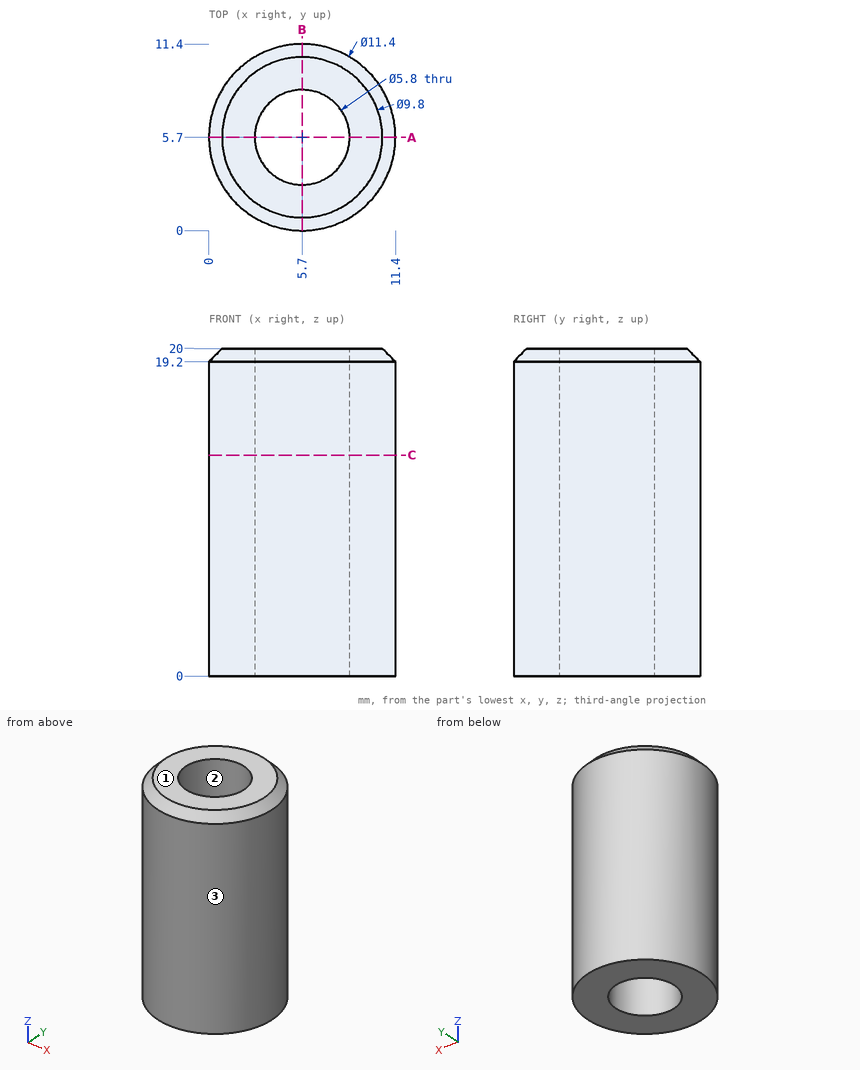
Check sheet for the drawn part. Datum: minimum x, y, z corner. Units: mm. Round coordinates to 2 decimals unless told otherwise and drop trailing zeros. Order: outer loops, then holes, each group sorted by start corner. A loop starts at its lowest first (then second) coordinate and runs counter-clockwise, first axis right, second up. Notation, with made-up numbers: M -0.5,-20 L 24.5,-20 A26 ccw 24.5,2 Z; hole C -3,40.5 d3. An arc over 180 degrees is marked long. Answer in a Markdown table with one row per item.
(1) Section check C-C on z = 13.5. Record the boundary of the cut face in (x, y).
Findings:
| item | result |
|---|---|
| outline | C 5.7,5.7 d11.4; hole C 5.7,5.7 d5.8 |
(2) Draft check along Y on the marked faces 1, 2 and 3. Enter one of: +Y half, -Y half, draft (parallel to the pull), parting line (faces both ways), or undercut.
Findings:
| item | result |
|---|---|
| face 1 | draft |
| face 2 | undercut |
| face 3 | parting line |
(3) Section check A-A on y = 5.7. Record the boundary of the cut face in (x, z).
Findings:
| item | result |
|---|---|
| outline | M 0,0 L 2.8,0 L 2.8,20 L 0.8,20 L 0,19.2 Z; M 8.6,0 L 11.4,0 L 11.4,19.2 L 10.6,20 L 8.6,20 Z |
(4) Material ranges on line 1 along Y through (x, z) = (5.7, 9.25); line 2 along X through (y, z) = (7.25, 15.25); line 3 along X through (y, z) = (5, 17.5), recorded low to high. Write a range as from..to.
Findings:
| item | result |
|---|---|
| line 1 | y = 0..2.8, 8.6..11.4 |
| line 2 | x = 0.21..3.25, 8.15..11.19 |
| line 3 | x = 0.04..2.89, 8.51..11.36 |
(5) Gauge pin test, flat ends, axial feed: pin 1 (4 mm diameter, centred on y = 10, z = 16, fed in from +X); pin 2 (1 mm diameter, centred on x = 9.5, y = 1.5, fed in from +Z); pin 3 (3 mm diameter, centred on y = 10, z = 15, fed in from -X). Record the tip position at first contact, or that the pin passes through.
Findings:
| item | result |
|---|---|
| pin 1 | stops at x = 10.92 |
| pin 2 | stops at z = 19.74 |
| pin 3 | stops at x = 0.74 |
